Answer from the drawing. Dimensions are ordinates in mm from the lowest x, y and z of the part. A direction names the side the tool comes from. Coordinates: 2 decimals unless noted, no trailing zeros. Write each loop counter-clockwise with the first axis right and the second up, starting at its lowest first coordinate (ties: lowest second). Pieces come first, ordered by that corner, then holes. Notation, with made-up numbers: (17.25, 62) - (72.25, 62) arc R33 cw to (72.25, 93) - close; hole circle Ø1 at (40.25, 84.25). An arc over 180 degrees is marked (long way). Return JSON: item names as keys, results as strings.
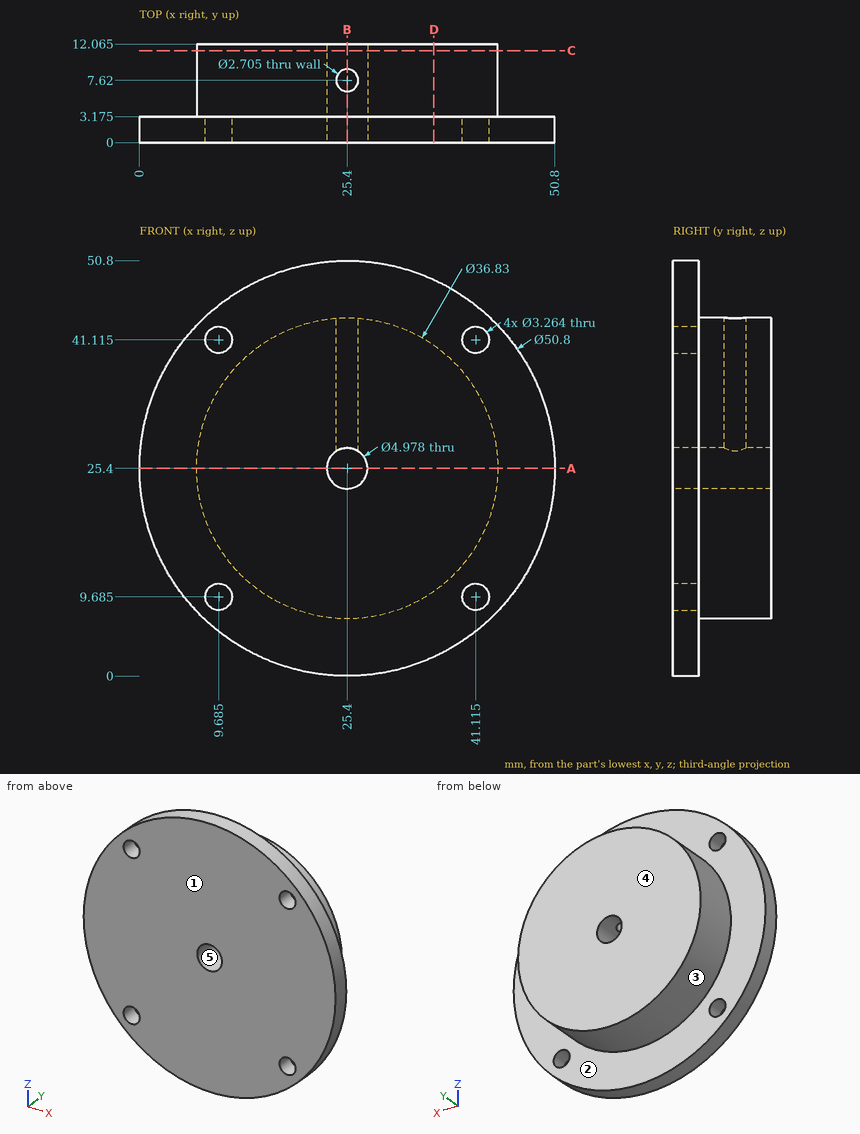
(1) Which of the six approach directions +Z, -Z, +X, -X, +Y, -Y give full straight-line access (tool end or side, diameter ignored) to the marked faces 1 and 2?
Answer:
{"face 1": "+Z, -Z, +X, -X, -Y", "face 2": "+Y"}
(2) Determine the mould class of the marked faces 3, 4 and 5 for opening direction Z: +Z half, -Z half, draft (parallel to the pull), parting line (faces both ways), or undercut.
Answer:
{"face 3": "parting line", "face 4": "draft", "face 5": "undercut"}
(3) Flat-ended cylindrical pins translate along their axes: P1, Ø2, axis at y = 10.5, z = 18.5, coming from the -X side (1 decimal); P2, Ø4.5, axis at x = 25.4, y = 7.62, coming from the +Z side (3 decimals); P3, Ø4, axis at x = 41.12, z = 9.68, coming from the +Y side (3 decimals). Find the tip coordinate at first contact, or state that the pin passes through.
Answer:
{"P1": "x = 8", "P2": "z = 43.815", "P3": "y = 3.175"}
(4) A cutting plane is placed at A-A (z = 25.4). Determine the outline of the cut face in (x, y) (1 decimal).
Answer:
{"outline": "(0, 0) - (22.9, 0) - (22.9, 12.1) - (7, 12.1) - (7, 3.2) - (0, 3.2) - close; (27.9, 0) - (50.8, 0) - (50.8, 3.2) - (43.8, 3.2) - (43.8, 12.1) - (27.9, 12.1) - close"}
(5) A cutting plane is placed at B-B (x = 25.4). Determine the outline of the cut face in (y, z) (1 decimal).
Answer:
{"outline": "(0, 0) - (3.2, 0) - (3.2, 7) - (12.1, 7) - (12.1, 22.9) - (0, 22.9) - close; (0, 27.9) - (6.3, 27.9) - (6.3, 43.8) - (3.2, 43.8) - (3.2, 50.8) - (0, 50.8) - close; (9, 27.9) - (12.1, 27.9) - (12.1, 43.8) - (9, 43.8) - close"}
(6) A cutting plane is placed at D-D (x = 36). Determine the outline of the cut face in (y, z) (1 decimal), and give its area (3 significant figures).
Answer:
{"outline": "(0, 2.3) - (3.2, 2.3) - (3.2, 10.3) - (12.1, 10.3) - (12.1, 40.5) - (3.2, 40.5) - (3.2, 48.5) - (0, 48.5) - close", "area": "414 mm²"}
(7) A cutting plane is placed at C-C (y = 11.25). Determine the outline of the cut face in (x, z) (1 decimal), and give its area (3 significant figures).
Answer:
{"outline": "circle Ø36.8 at (25.4, 25.4); hole circle Ø5 at (25.4, 25.4)", "area": "1,050 mm²"}
(8) Straight lines are drawn through the part: line 1 (Z direction, x = 25.5, y = 2.25); line 2 (Y direction, x = 25.4, z = 31.5) (1 decimal); line 3 (Y direction, x = 36.5, z = 43.5) (1 decimal). For each, find the intervals that lie inside material, in ascending order. Write a range as from..to.
Answer:
{"line 1": "0..22.91, 27.89..50.8", "line 2": "0..6.3, 9..12.1", "line 3": "0..3.2"}
